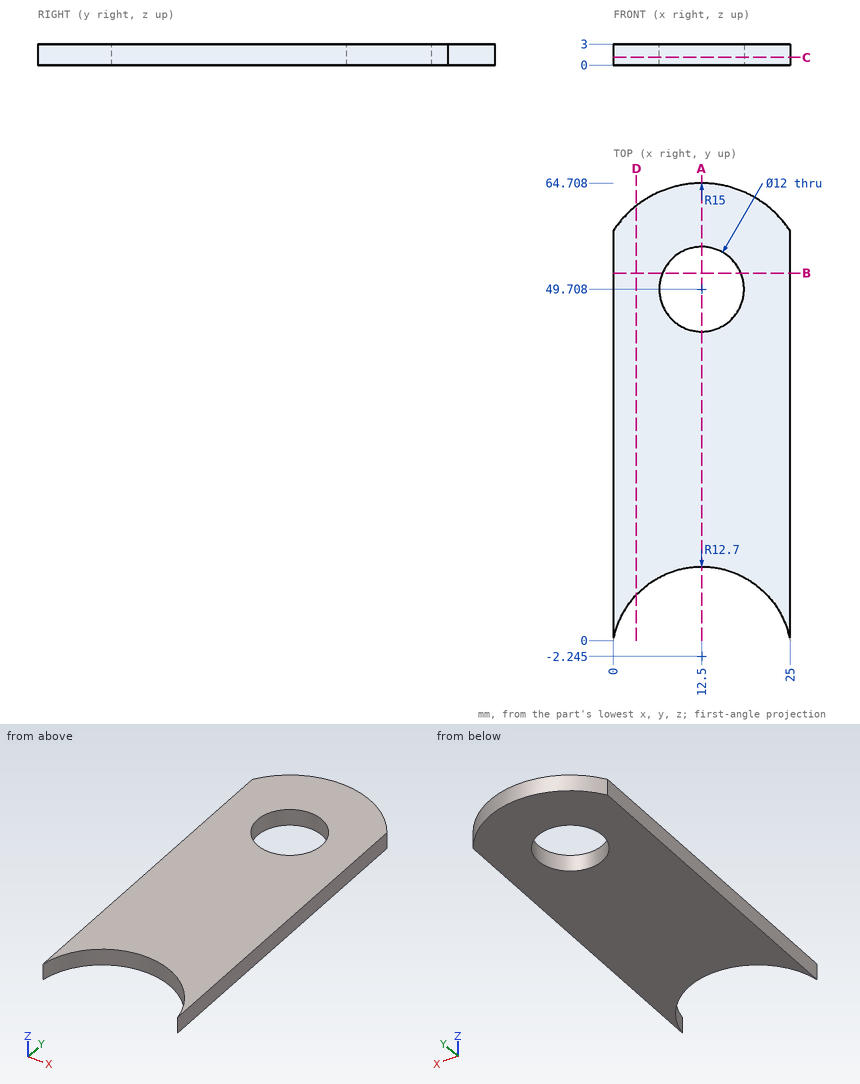
Print and shaded views of the part. All mm, measured from the part's lowest x, y and z. Coordinates: 2 decimals unless noted, no trailing zeros. Loops run counter-clockwise (first coordinate to the right, second up) from the corner with the lowest first, then second, coordinate; pieces in that order, holes last. Notation, with made-up numbers: M 29.25,3 L 41.25,3 A31 cw 41.25,40 Z; hole C 61.5,-8 d7. An arc over 180 degrees is marked long. Use a Markdown table: item, result. Add a question column.
Q1. Pin check, flat tips, straight feed: P1, Ø1, axis at x = 20, z = 2.5, coming from the -Y side; P2, Ø11, axis at x = 12.5, y = 49.71, coming from the -Z side. Stop position of each tip, or through.
Q2. Probe L1, parallel to X at y = 49.5, z = 1.8; L2, parallel to X at y = 51.5, z = 2.6 (1 decimal); L3, parallel to Y at x = 10.75, z = 0.2 (1 decimal). List the from-to ranges inside material, lowest first.
Q3. Cut at C-C (z = 1.1). Write the cut outline in (x, y) (1 decimal).
Q4. Cut at B-B (y = 52). Write the cut outline in (x, z) (1 decimal).
Q5. Cut at A-A (x = 12.5). Write the cut outline in (y, z) (1 decimal).
Q6. Cut at D-D (x = 3.25). Write the cut outline in (y, z).
Worked out:
| question | item | result |
|---|---|---|
| 1 | P1 | stops at y = 7.62 |
| 1 | P2 | passes through |
| 2 | L1 | x = 0 to 6.5, 18.5 to 25 |
| 2 | L2 | x = 0 to 6.8, 18.2 to 25 |
| 2 | L3 | y = 10.3 to 44, 55.4 to 64.6 |
| 3 | outline | M 0,0 A12.7 cw 25,0 L 25,58 A15 ccw 0,58 Z; hole C 12.5,49.7 d12 |
| 4 | outline | M 0,0 L 7,0 L 7,3 L 0,3 Z; M 18,0 L 25,0 L 25,3 L 18,3 Z |
| 5 | outline | M 10.5,0 L 43.7,0 L 43.7,3 L 10.5,3 Z; M 55.7,0 L 64.7,0 L 64.7,3 L 55.7,3 Z |
| 6 | outline | M 6.46,0 L 61.52,0 L 61.52,3 L 6.46,3 Z |
